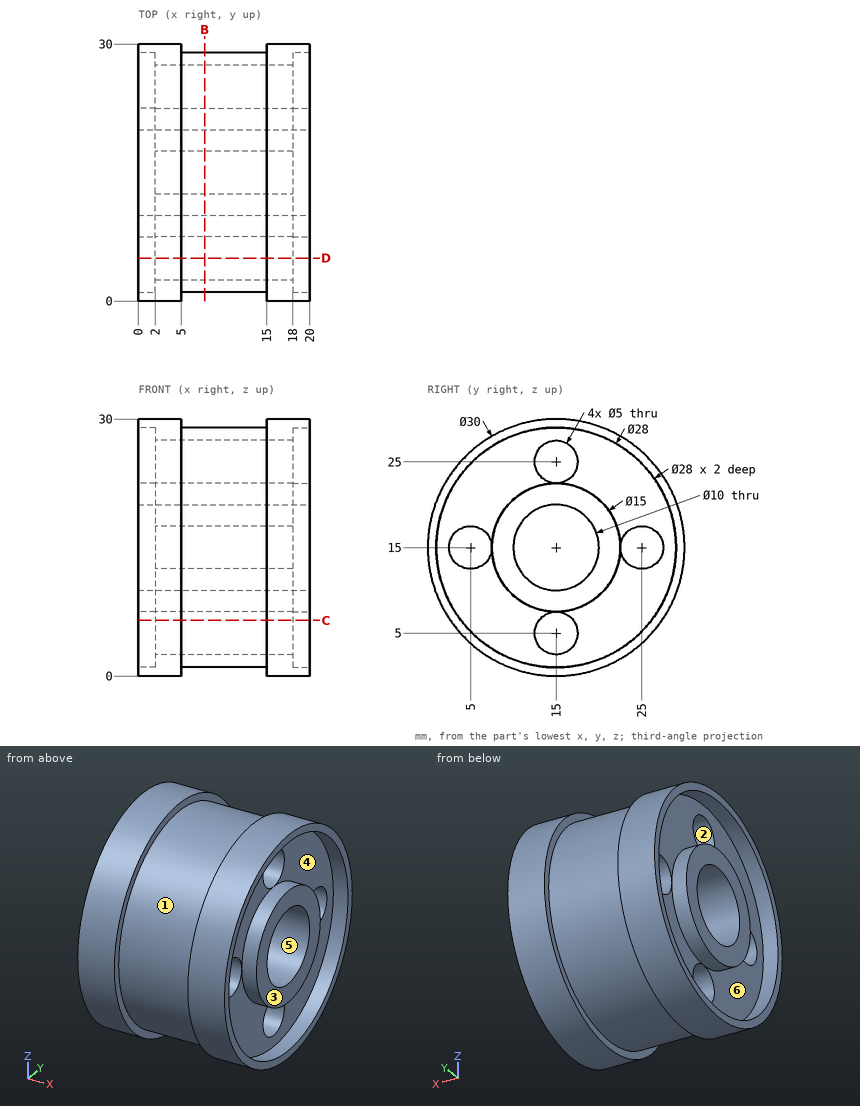
Print and shaded views of the part. All mm, measured from the part's lowest x, y and z. A direction names the side the tool comes from. Coordinates: 2 decimals unless noted, no trailing zeros. Loops run counter-clockwise (first coordinate to the right, second up) from the corner with the lowest first, then second, coordinate; pieces in that order, holes last. Notation, with made-up numbers: (67.5, -36.5) -> (90.5, -36.5) arc R23 cw to (90.5, -13.5) -> close; hole circle Ø6 at (51.25, -16.5). An arc over 180 degrees is marked (long way). Use one line per item in the form item = value. Start each with the question number.
(1) Pull direction Z, two halves, no side cores. Call the marked faces 1, 2 and 3: pulls with the +Z half, pulls with the -Z half, needs draft (parallel to the pull), parting line crosses it, or undercut.
(2) Flat gauge pins, fed straight in: pin 1 (2 mm diameter, centred on x = 17.5, z = 12.5, fed in from +Y); pin 2 (1.5 mm diameter, centred on x = 8.5, y = 3, fed in from +Z); pin 3 (3 mm diameter, centred on x = 16, z = 7.5, fed in from +Y). Where does each tip first touch, or does it go through?
(3) Cut at D-D on y = 5. Give the cut face in (x, z), and give its area (3 significant figures).
(4) Probe probe 1 along Z at (x, y) = (12.5, 15); probe 2 along Z at (x, y) = (0.5, 15); probe 3 along X at (y, z) = (25.25, 19.25). List the from-to ranges inside material, lowest first. Write a range as from..to.
(5) Cut at C-C on z = 6.5. Give the cut face in (x, y), and give its area (3 significant figures).
(6) Cut at B-B on x = 7.75. Give the cut face in (y, z).
(7) Tool access for the marked faces 4, 5 and 6: list every direction of +Z, -Z, +X, -X, +Y, -Y with a clear straight run to the whole face (end or side of a thin tool).
Values:
q1.face_1 = parting line crosses it
q1.face_2 = undercut
q1.face_3 = needs draft
q2.pin_1 = 29.92
q2.pin_2 = 23.33
q2.pin_3 = 28.75
q3.outline = (0, 3.82) -> (5, 3.82) -> (5, 5.2) -> (15, 5.2) -> (15, 3.82) -> (20, 3.82) -> (20, 5.2) -> (18, 5.2) -> (18, 12.5) -> (2, 12.5) -> (2, 5.2) -> (0, 5.2) -> close; (0, 24.8) -> (2, 24.8) -> (2, 17.5) -> (18, 17.5) -> (18, 24.8) -> (20, 24.8) -> (20, 26.18) -> (15, 26.18) -> (15, 24.8) -> (5, 24.8) -> (5, 26.18) -> (0, 26.18) -> close
q3.area = 261 mm2
q4.probe_1 = 1..2.5, 7.5..10, 20..22.5, 27.5..29
q4.probe_2 = 0..1, 7.5..10, 20..22.5, 29..30
q4.probe_3 = 2..18
q5.outline = (0, 2.64) -> (5, 2.64) -> (5, 3.88) -> (15, 3.88) -> (15, 2.64) -> (20, 2.64) -> (20, 3.88) -> (18, 3.88) -> (18, 13) -> (2, 13) -> (2, 3.88) -> (0, 3.88) -> close; (0, 26.12) -> (2, 26.12) -> (2, 17) -> (18, 17) -> (18, 26.12) -> (20, 26.12) -> (20, 27.36) -> (15, 27.36) -> (15, 26.12) -> (5, 26.12) -> (5, 27.36) -> (0, 27.36) -> close
q5.area = 317 mm2
q6.outline = circle Ø28 at (15, 15); hole circle Ø5 at (5, 15); hole circle Ø10 at (15, 15); hole circle Ø5 at (15, 5); hole circle Ø5 at (15, 25); hole circle Ø5 at (25, 15)
q7.face_4 = +X
q7.face_5 = +X, -X
q7.face_6 = -X
